Source: CAD feature listing. Evaluate the final solid. Frame: model axes, mm. Face numbers are marked on the shaded views. A direction names the side the tool comes from. Give positions to 0.01 mm unless a question says otherwise; leave off trailing zeros. Loops run counter-clockwise (first coordinate to the right, second up) from the corner with the lowest first, then second, coordinate; pieces in that order, holes last. Notation, with made-up numbers: M 48.25,28 L 79.25,28 A25 cw 79.25,57 Z; hole C 8.5,76 d5. An arc over 180 degrees is marked long. Answer in a Markdown table with one row per item.
```python
from build123d import *

# Parameters (mm, degrees)
F2_DEPTH = 11.684
F3_W     = 23.6796867102
F3_H     = 69.1230408847
F4_DEPTH = 25.4
F5_DEPTH = 102.108
F7_DEPTH = 25.4
F8_DEPTH = 110.49


with BuildPart() as f2:
    # F0 (on Top) → F2 (new body)
    with BuildSketch(Plane.XY):
        with BuildLine():
            Line((-39.3080597717, -40.7505296171), (20.7232069224, -40.7505296171))
            Line((20.7232069224, -40.7505296171), (20.7232069224, -28.3725112677))
            Line((20.7232069224, -28.3725112677), (44.4028936327, -28.3725112677))
            Line((44.4028936327, -28.3725112677), (44.4028936327, 40.7505296171))
            Line((44.4028936327, 40.7505296171), (-39.3080597717, 40.7505296171))
            ThreePointArc((-39.3080597717, 40.7505296171), (-85.4706790142, 0), (-39.3080597717, -40.7505296171))
        make_face()
    extrude(amount=F2_DEPTH)

    # F3 (on face) → F4 (join)
    with BuildSketch(Plane.XY.offset(11.684)):
        with Locations((32.5630502775, 6.1890091747)):
            Rectangle(F3_W, F3_H)
    extrude(amount=F4_DEPTH)

    # F5 (add): a face of the model
    f5_faces = [f2.faces().sort_by_distance(p)[0] for p in [
        (32.5630502775, 6.1890091747, 37.084),
    ]]
    extrude(f5_faces, amount=F5_DEPTH)

    # F6 (on face) → F7 (join)
    with BuildSketch(Plane(origin=(20.7232069224, 0, 0), x_dir=(0, -1, 0), z_dir=(-1, 0, 0))):
        with BuildLine():
            Line((1.971335616, 139.192), (-17.6932327449, 139.192))
            Line((-17.6932327449, 139.192), (-17.6932327449, 46.8966588378))
            Line((-17.6932327449, 46.8966588378), (-17.4947245486, 46.8966588378))
            ThreePointArc((-17.4947245486, 46.8966588378), (-7.8609485645, 37.2628828536), (1.7728274197, 46.8966588378))
            Line((1.7728274197, 46.8966588378), (1.971335616, 46.8966588378))
            Line((1.971335616, 46.8966588378), (1.971335616, 139.192))
        make_face()
    extrude(amount=F7_DEPTH)

    # F8 (cut): a face of the model
    f8_faces = [f2.faces().sort_by_distance(p)[0] for p in [
        (-4.6767930776, 7.8609485645, 89.3091389319),
    ]]
    extrude(f8_faces, amount=-F8_DEPTH, mode=Mode.SUBTRACT)


solid = f2.part
```
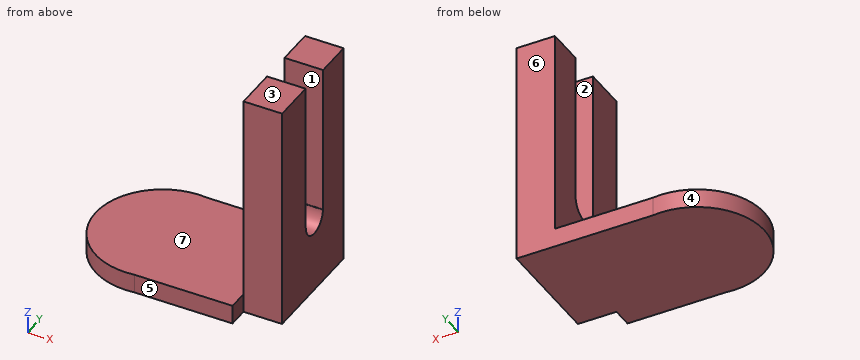
1) Section B-B, the plane z = 9. Return loops of the section in (x, y).
Reply:
| item | result |
|---|---|
| outline | M -39.31,-40.75 L 20.72,-40.75 L 20.72,-28.37 L 44.4,-28.37 L 44.4,40.75 L -39.31,40.75 A41.07 ccw long Z |
2) Pull-direction query (Y, two-part tool) for the marked faces 1, 2, 3 and 4; classes: released by +Y, released by -Y, zero draft, split by the parting line, or undercut.
Reply:
| item | result |
|---|---|
| face 1 | undercut |
| face 2 | undercut |
| face 3 | zero draft |
| face 4 | split by the parting line |
3) Material intervals for L1, parallel to Z at x = 39.5, y = 8.5; L2, parallel to Z at x = -58, y = 10.5; L3, parallel to X at y = 26, z = 118.5, sorted ascending.
Reply:
| item | result |
|---|---|
| L1 | z = 0 to 37.28 |
| L2 | z = 0 to 11.68 |
| L3 | x = 20.72 to 44.4 |
4) Section C-C, the plane x = -5.5. Return loops of the section in (y, z), then the cut area to 3 significant figures.
Reply:
| item | result |
|---|---|
| outline | M -40.75,0 L 40.75,0 L 40.75,11.68 L -40.75,11.68 Z |
| area | 952 mm² |
5) Set-up query: the marked faces 5, 6 and 7. Return all of +Z, -Z, +X, -X, +Y, -Y with unobstructed straight access to the full face (end or side cutting, diameter ignored); none if empty.
Reply:
| item | result |
|---|---|
| face 5 | +Z, -Z, +X, -Y |
| face 6 | +Z, -Z, +X, +Y |
| face 7 | +Z, -X, +Y, -Y |
6) Section D-D, the plane y = 26.5. Return loops of the section in (x, z).
Reply:
| item | result |
|---|---|
| outline | M -75.78,0 L 44.4,0 L 44.4,139.19 L 20.72,139.19 L 20.72,11.68 L -75.78,11.68 Z |
7) Pin query (flat end, axial travel): pin 1 Ø1 at (y, z) = (28.5, 95) entering from -X; pin 2 Ø9.5 at (y, z) = (-37.5, 7.5) entering from +X; pin 3 Ø4 at (x, z) = (26, 74) entering from -Y; pin 4 Ø3 at (x, y) = (-71.5, -21) entering from -Z. Return the tip coordinate at first contact, or that it passes through.
Reply:
| item | result |
|---|---|
| pin 1 | stops at x = 20.72 |
| pin 2 | stops at x = 20.72 |
| pin 3 | stops at y = -28.37 |
| pin 4 | stops at z = 0 |
8) Section A-A, the plane z = 105. Return loops of the section in (x, y).
Reply:
| item | result |
|---|---|
| outline | M 20.72,-28.37 L 44.4,-28.37 L 44.4,-1.97 L 20.72,-1.97 Z; M 20.72,17.69 L 44.4,17.69 L 44.4,40.75 L 20.72,40.75 Z |
